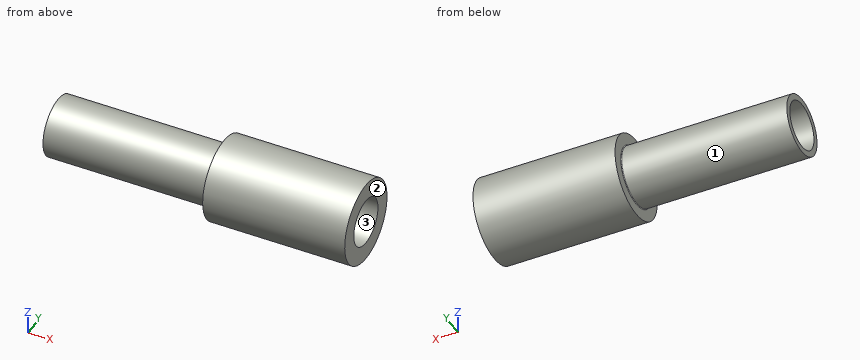
```python
from build123d import *

# Parameters (mm, degrees)
SZKIC1_R                    = 12.5
SZKIC1_R_2                  = 10
DODANIE_WYCI_GNI_CIE1_DEPTH = 70
SZKIC2_R                    = 17.5
SZKIC2_R_2                  = 10
DODANIE_WYCI_GNI_CIE2_DEPTH = 60
ZAOKR_GLENIE1_R             = 0.3


with BuildPart() as part:
    # Szkic1 → Dodanie-wyciągnięcie1 (new body)
    with BuildSketch(Plane(origin=(0, 0, 0), x_dir=(0, 0, -1), z_dir=(1, 0, 0))):
        Circle(SZKIC1_R)
        Circle(SZKIC1_R_2, mode=Mode.SUBTRACT)
    extrude(amount=DODANIE_WYCI_GNI_CIE1_DEPTH)

    # Szkic2 → Dodanie-wyciągnięcie2 (add)
    with BuildSketch(Plane(origin=(70, 0, 0), x_dir=(0, 0, -1), z_dir=(1, 0, 0))):
        Circle(SZKIC2_R)
        Circle(SZKIC2_R_2, mode=Mode.SUBTRACT)
    extrude(amount=DODANIE_WYCI_GNI_CIE2_DEPTH)

    # Zaokrąglenie1
    zaokr_glenie1_edges = [part.edges().sort_by_distance(p)[0] for p in [
        (70, 0, 12.5),
    ]]
    fillet(zaokr_glenie1_edges, radius=ZAOKR_GLENIE1_R)


solid = part.part
```
Read the model definition and answer for the solid it produces. Units are mm, in the model's axes. Face numbers are marked on the shaded views. Give positions to 0.01 mm unless a question says otherwise; leave off trailing zeros. Write each loop counter-clockwise with the first axis right and the second up, starting at its lowest first coordinate (ties: lowest second). Pieces come first, ordered by that corner, then holes. Notation, with made-up numbers: M 35.25,44 L 42.25,44 A12 cw 42.25,52 Z; hole C 22,51.25 d2. An arc over 180 degrees is marked long. Put each result on its own line as item: value. Start each with the question number.
1. The part is cut by section A-A, the plane y = 0. Give the vertices of the cut face in (x, z).
2. The part is cut by section C-C, the plane x = 116.5. Give the vertices of the cut face in (y, z).
3. The part is cut by section D-D, the plane x = 19.5. Give the vertices of the cut face in (y, z).
4. Consider line 1 along Y through (x, z) = (42, -0.5); line 2 along Y through (x, z) = (80.5, 0); line 3 along X through (y, z) = (15, -1). Determine where each line is inside the solid, lowest interval first.
5. Each of these flat-tipped pins is pushed along its axis until it touches: pin 1 Ø5 at (x, y) = (26, 0) entering from +Z; pin 2 Ø4 at (x, y) = (89, -3.5) entering from +Z; pin 3 Ø2 at (x, y) = (16.5, 8) entering from -Z; pin 4 Ø18 at (y, z) = (0, 0) entering from +X. Where does it stop, or does it pass through?
6. For a pull along Z with two mould halves and no side action, classify the marked faces 1, 2 and 3 as released by +Z, released by -Z, zero draft, split by the parting line, or undercut.
Final values:
1. outline: M 0,-12.5 L 69.7,-12.5 A0.3 cw 70,-12.8 L 70,-17.5 L 130,-17.5 L 130,-10 L 0,-10 Z; M 0,10 L 130,10 L 130,17.5 L 70,17.5 L 70,12.8 A0.3 cw 69.7,12.5 L 0,12.5 Z
2. outline: C 0,0 d35; hole C 0,0 d20
3. outline: C 0,0 d25; hole C 0,0 d20
4. line 1: y = -12.49 to -9.99, 9.99 to 12.49
4. line 2: y = -17.5 to -10, 10 to 17.5
4. line 3: x = 70 to 130
5. pin 1: stops at z = 12.5
5. pin 2: stops at z = 17.44
5. pin 3: stops at z = -10.36
5. pin 4: passes through
6. face 1: split by the parting line
6. face 2: zero draft
6. face 3: undercut
